The figure shows three views and two pictorial views of one solid part (mm, origin at its lowest corner). Answer the questions. A direction names the side the tool comes from. Give positions to 0.01 mm unless a question says otherwise; leave off trailing zeros. Write each loop counter-clockwise with the first axis right and the second up, starting at its lowest first coordinate (ties: lowest second). Pieces come first, ordered by that corner, then holes. Notation, with made-up numbers: M 41,-40 L 82,-40 A28 ccw 82,-12 Z; hole C -26.5,32 d7. An arc over 180 degrees is marked long. Return JSON: item names as keys, results as strings.
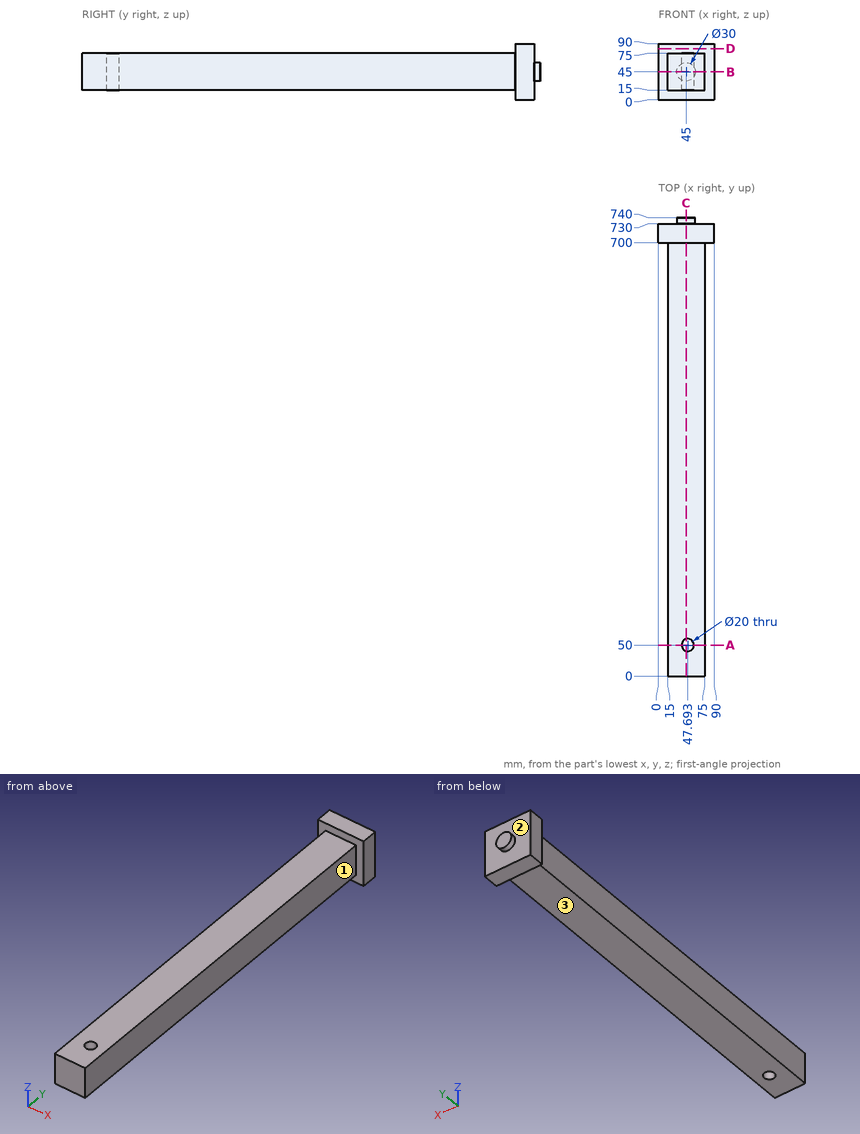
Item 1: Which of the six approach directions +Z, -Z, +X, -X, +Y, -Y give full straight-line access (tool end or side, diameter ignored) to the marked faces 1, 2 and 3?
Geometry results:
{"face 1": "+Z, -Z, +X, -Y", "face 2": "+Y", "face 3": "-Z, +X, -X, -Y"}
Item 2: A cutting plane is placed at C-C, the plane x = 45. Write down the section's boundary in (y, z).
Geometry results:
{"outline": "M 0,15 L 40.37,15 L 40.37,75 L 0,75 Z; M 59.63,15 L 700,15 L 700,0 L 730,0 L 730,30 L 740,30 L 740,60 L 730,60 L 730,90 L 700,90 L 700,75 L 59.63,75 Z"}
Item 3: Find the intervals of material crossed by line 1 (X direction, y = 50, z = 48); line 2 (Y direction, x = 47, z = 39); line 3 (X direction, y = 299.5, z = 64.5), in increasing order.
Geometry results:
{"line 1": "x = 15 to 37.69, 57.69 to 75", "line 2": "y = 0 to 40.02, 59.98 to 740", "line 3": "x = 15 to 75"}
Item 4: A cutting plane is placed at B-B, the plane z = 45. Write down the section's boundary in (x, y), plus the area to 3 significant figures.
Geometry results:
{"outline": "M 0,700 L 15,700 L 15,0 L 75,0 L 75,700 L 90,700 L 90,730 L 60,730 L 60,740 L 30,740 L 30,730 L 0,730 Z; hole C 47.69,50 d20", "area": "44,700 mm2"}
Item 5: Given pin 1 Ø3 at (x, z) = (48.5, 20) entering from -Y; pin 2 Ø18 at (y, z) = (400.5, 32) entering from -X; pin 3 Ø4 at (x, y) = (35.5, 445) entering from +Z; pin 4 Ø2 at (x, z) = (15, 56.5) entering from +Y, each flat-ended and moving along its own axis, determine where each tip first touches the part or whether it passes through.
Geometry results:
{"pin 1": "stops at y = 0", "pin 2": "stops at x = 15", "pin 3": "stops at z = 75", "pin 4": "stops at y = 730"}
Item 6: A cutting plane is placed at A-A, the plane y = 50. Write down the section's boundary in (x, z), plus the area to 3 significant figures.
Geometry results:
{"outline": "M 15,15 L 37.69,15 L 37.69,75 L 15,75 Z; M 57.69,15 L 75,15 L 75,75 L 57.69,75 Z", "area": "2,400 mm2"}
Item 7: A cutting plane is placed at D-D, the plane z = 82.5. Write down the section's boundary in (x, y).
Geometry results:
{"outline": "M 0,700 L 90,700 L 90,730 L 0,730 Z"}
